Work out the finished part from the listing and answer in its coordinate system (mm). Face numbers are marked on the shaded views. A direction names the side the tool comes from. Coordinates: 2 decimals unless noted, no trailing zeros. Write each loop counter-clockwise with the first axis right and the second up, starting at its lowest first coordinate (ties: lowest second). Pieces come first, ordered by that corner, then holes. Notation, with made-up numbers: M 2.5,4.5 L 38.5,4.5 A23 ccw 38.5,27.5 Z; hole C 27,44 d7. An arc over 180 degrees is marked long. Use CSV: the item, a comma, the result in double quotes.
from build123d import *

# Parameters (mm, degrees)
BOSS_EXTRUDE1_DEPTH = 4
SKETCH3_R           = 12.5
BOSS_EXTRUDE2_DEPTH = 2
BOSS_EXTRUDE3_START = 2
SKETCH4_R           = 12.5
BOSS_EXTRUDE3_DEPTH = 2
SKETCH5_R           = 3
BOSS_EXTRUDE4_DEPTH = 10
SKETCH6_R           = 5
SKETCH6_R_2         = 3
BOSS_EXTRUDE5_DEPTH = 2


with BuildPart() as part:
    # Sketch2 → Boss-Extrude1 (new body)
    with BuildSketch(Plane.XY):
        with BuildLine():
            Line((0, 9.5), (-0.977834373, 7.940015109))
            ThreePointArc((-0.977834373, 7.940015109), (-1.25147572, 7.901506725), (-1.523623852, 7.853570548))
            Line((-1.523623852, 7.853570548), (-2.935661447, 9.035036905))
            Line((-2.935661447, 9.035036905), (-3.383575357, 7.24923567))
            ThreePointArc((-3.383575357, 7.24923567), (-3.631923998, 7.128052194), (-3.875939159, 6.998363783))
            Line((-3.875939159, 6.998363783), (-5.583959897, 7.685661447))
            Line((-5.583959897, 7.685661447), (-5.45810841, 5.848850535))
            ThreePointArc((-5.45810841, 5.848850535), (-5.656854249, 5.656854249), (-5.848850535, 5.45810841))
            Line((-5.848850535, 5.45810841), (-7.685661447, 5.583959897))
            Line((-7.685661447, 5.583959897), (-6.998363783, 3.875939159))
            ThreePointArc((-6.998363783, 3.875939159), (-7.128052194, 3.631923998), (-7.24923567, 3.383575357))
            Line((-7.24923567, 3.383575357), (-9.035036905, 2.935661447))
            Line((-9.035036905, 2.935661447), (-7.853570548, 1.523623852))
            ThreePointArc((-7.853570548, 1.523623852), (-7.901506725, 1.25147572), (-7.940015109, 0.977834373))
            Line((-7.940015109, 0.977834373), (-9.5, 0))
            Line((-9.5, 0), (-7.940015109, -0.977834373))
            ThreePointArc((-7.940015109, -0.977834373), (-7.901506725, -1.25147572), (-7.853570548, -1.523623852))
            Line((-7.853570548, -1.523623852), (-9.035036905, -2.935661447))
            Line((-9.035036905, -2.935661447), (-7.24923567, -3.383575357))
            ThreePointArc((-7.24923567, -3.383575357), (-7.128052194, -3.631923998), (-6.998363783, -3.875939159))
            Line((-6.998363783, -3.875939159), (-7.685661447, -5.583959897))
            Line((-7.685661447, -5.583959897), (-5.848850535, -5.45810841))
            ThreePointArc((-5.848850535, -5.45810841), (-5.656854249, -5.656854249), (-5.45810841, -5.848850535))
            Line((-5.45810841, -5.848850535), (-5.583959897, -7.685661447))
            Line((-5.583959897, -7.685661447), (-3.875939159, -6.998363783))
            ThreePointArc((-3.875939159, -6.998363783), (-3.631923998, -7.128052194), (-3.383575357, -7.24923567))
            Line((-3.383575357, -7.24923567), (-2.935661447, -9.035036905))
            Line((-2.935661447, -9.035036905), (-1.523623852, -7.853570548))
            ThreePointArc((-1.523623852, -7.853570548), (-1.25147572, -7.901506725), (-0.977834373, -7.940015109))
            Line((-0.977834373, -7.940015109), (0, -9.5))
            Line((0, -9.5), (0.977834373, -7.940015109))
            ThreePointArc((0.977834373, -7.940015109), (1.25147572, -7.901506725), (1.523623852, -7.853570548))
            Line((1.523623852, -7.853570548), (2.935661447, -9.035036905))
            Line((2.935661447, -9.035036905), (3.383575357, -7.24923567))
            ThreePointArc((3.383575357, -7.24923567), (3.631923998, -7.128052194), (3.875939159, -6.998363783))
            Line((3.875939159, -6.998363783), (5.583959897, -7.685661447))
            Line((5.583959897, -7.685661447), (5.45810841, -5.848850535))
            ThreePointArc((5.45810841, -5.848850535), (5.656854249, -5.656854249), (5.848850535, -5.45810841))
            Line((5.848850535, -5.45810841), (7.685661447, -5.583959897))
            Line((7.685661447, -5.583959897), (6.998363783, -3.875939159))
            ThreePointArc((6.998363783, -3.875939159), (7.128052194, -3.631923998), (7.24923567, -3.383575357))
            Line((7.24923567, -3.383575357), (9.035036905, -2.935661447))
            Line((9.035036905, -2.935661447), (7.853570548, -1.523623852))
            ThreePointArc((7.853570548, -1.523623852), (7.901506725, -1.25147572), (7.940015109, -0.977834373))
            Line((7.940015109, -0.977834373), (9.5, 0))
            Line((9.5, 0), (7.940015109, 0.977834373))
            ThreePointArc((7.940015109, 0.977834373), (7.901506725, 1.25147572), (7.853570548, 1.523623852))
            Line((7.853570548, 1.523623852), (9.035036905, 2.935661447))
            Line((9.035036905, 2.935661447), (7.24923567, 3.383575357))
            ThreePointArc((7.24923567, 3.383575357), (7.128052194, 3.631923998), (6.998363783, 3.875939159))
            Line((6.998363783, 3.875939159), (7.685661447, 5.583959897))
            Line((7.685661447, 5.583959897), (5.848850535, 5.45810841))
            ThreePointArc((5.848850535, 5.45810841), (5.656854249, 5.656854249), (5.45810841, 5.848850535))
            Line((5.45810841, 5.848850535), (5.583959897, 7.685661447))
            Line((5.583959897, 7.685661447), (3.875939159, 6.998363783))
            ThreePointArc((3.875939159, 6.998363783), (3.631923998, 7.128052194), (3.383575357, 7.24923567))
            Line((3.383575357, 7.24923567), (2.935661447, 9.035036905))
            Line((2.935661447, 9.035036905), (1.523623852, 7.853570548))
            ThreePointArc((1.523623852, 7.853570548), (1.25147572, 7.901506725), (0.977834373, 7.940015109))
            Line((0.977834373, 7.940015109), (0, 9.5))
        make_face()
    extrude(amount=BOSS_EXTRUDE1_DEPTH)

    # Sketch3 → Boss-Extrude2 (add)
    with BuildSketch(Plane.XY.offset(4)):
        Circle(SKETCH3_R)
    extrude(amount=BOSS_EXTRUDE2_DEPTH)

    # Sketch4 → Boss-Extrude3 (add)
    with BuildSketch(Plane(origin=(0, 0, 0), x_dir=(-1, 0, 0), z_dir=(0, 0, -1)).offset(BOSS_EXTRUDE3_START)):
        with Locations(Location((0, 0, 0), (0, 0, 180))):
            Circle(SKETCH4_R)
    extrude(amount=-BOSS_EXTRUDE3_DEPTH)

    # Sketch5 → Boss-Extrude4 (add)
    with BuildSketch(Plane(origin=(0, 0, -2), x_dir=(-1, 0, 0), z_dir=(0, 0, -1))):
        Circle(SKETCH5_R)
    extrude(amount=BOSS_EXTRUDE4_DEPTH)

    # Sketch6 → Boss-Extrude5 (add)
    with BuildSketch(Plane(origin=(0, 0, -2), x_dir=(-1, 0, 0), z_dir=(0, 0, -1))):
        Circle(SKETCH6_R)
        Circle(SKETCH6_R_2, mode=Mode.SUBTRACT)
    extrude(amount=BOSS_EXTRUDE5_DEPTH)


solid = part.part
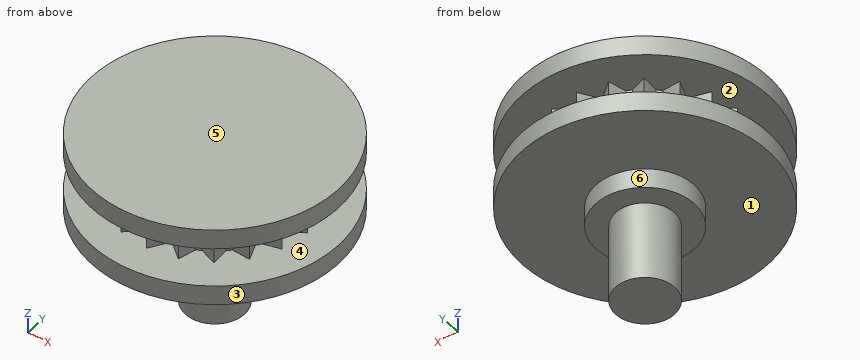
Item 1: The part is cut by section B-B (y = -4.5). Write down the section's boundary in (x, z), then the cut area to 3 significant figures.
Answer:
outline,"M -11.66,-2 L -2.18,-2 L -2.18,-4 L 2.18,-4 L 2.18,-2 L 11.66,-2 L 11.66,0 L 7.25,0 L 7.25,4 L 11.66,4 L 11.66,6 L -11.66,6 L -11.66,4 L -7.25,4 L -7.25,0 L -11.66,0 Z"
area,"160 mm2"
Item 2: The part is cut by section D-D (y = 4.25). Write down the section's boundary in (x, z).
Answer:
outline,"M -11.76,-2 L -2.63,-2 L -2.63,-4 L 2.63,-4 L 2.63,-2 L 11.76,-2 L 11.76,0 L 7.15,0 L 7.15,4 L 11.76,4 L 11.76,6 L -11.76,6 L -11.76,4 L -7.15,4 L -7.15,0 L -11.76,0 Z"
Item 3: The part is cut by section A-A (x = -10.25). Write down the section's boundary in (y, z).
Answer:
outline,"M -7.15,-2 L 7.15,-2 L 7.15,0 L -7.15,0 Z; M -7.15,4 L 7.15,4 L 7.15,6 L -7.15,6 Z"
Item 4: Consider probe 1 along Z at (x, y) = (7.25, -7.75); probe 2 along Z at (x, y) = (3.25, 1.5); probe 3 along X at (y, z) = (-0.75, -4.5). Determine where each line is inside the solid, lowest interval first.
Answer:
probe 1,"z = -2 to 0, 4 to 6"
probe 2,"z = -4 to 6"
probe 3,"x = -2.9 to 2.9"
Item 5: The part is cut by section C-C (z = 4.75). Write down the section's boundary in (x, y).
Answer:
outline,"C 0,0 d25"
Item 6: For a pull along Z with two mould halves and no side action, classify the marked faces 1, 2 and 3 as released by +Z, released by -Z, zero draft, split by the parting line, or undercut.
Answer:
face 1,"released by -Z"
face 2,"undercut"
face 3,"zero draft"
Item 7: Given pin 1 (1.5 mm diameter, centred on x = -2, z = 1.5, fed in from -Y); pin 2 (2 mm diameter, centred on y = 0, z = 2.5, fed in from -X); pin 3 (1.5 mm diameter, centred on x = 8.5, y = -4, fed in from -Z), each flat-ended and moving along its own axis, determine where each tip first touches the part or whether it passes through.
Answer:
pin 1,"stops at y = -8.88"
pin 2,"stops at x = -9.5"
pin 3,"stops at z = -2"
Item 8: A tool of negligible diameter and unlimited length cuts with its end or side. For the marked faces 4, 5 and 6, from which of +Z, -Z, +X, -X, +Y, -Y can it reach the whole face along a straight path? Write none if from no direction.
Answer:
face 4,"none"
face 5,"+Z, +X, -X, +Y, -Y"
face 6,"-Z"
